The listing builds one solid part. Answer for the finished solid, in the listing's coordinates (mm). Coordinates: 2 decimals unless noted, no trailing zeros. Loops run counter-clockwise (first coordinate to the right, second up) from the corner with the lowest first, then second, coordinate; pieces in that order, holes last. Notation, with made-up numbers: M 56,54 L 66,54 A23 cw 66,71 Z; hole C 30.25,-39 d1. An arc over 180 degrees is marked long. Answer in a Markdown table with one row per item. Add a question column.
from build123d import *

# Parameters (mm, degrees)
SKETCH4_R          = 100
CUT_EXTRUDE2_DEPTH = 10
SKETCH5_R          = 250
CUT_EXTRUDE4_DEPTH = 1
SKETCH6_R          = 1.241785282
CUT_EXTRUDE5_DEPTH = 201


with BuildPart() as part:
    # Sketch1 → Revolve2 (revolve)
    with BuildSketch(Plane.XY):
        Polygon((0, 0), (0, 251), (202, 251), (202, 150), align=None)
        Polygon((201, 249.758214718), (201, 151), (0.5, 2.113861386), (1, 249.758214718), align=None, mode=Mode.SUBTRACT)
    revolve(axis=Axis((0, 251, 0), (1, 0, 0)))

    # Sketch4 → Cut-Extrude2 (cut)
    with BuildSketch(Plane(origin=(202, 0, 0), x_dir=(0, 0, -1), z_dir=(1, 0, 0))):
        with Locations((0, 251)):
            Circle(SKETCH4_R)
    extrude(amount=-CUT_EXTRUDE2_DEPTH, mode=Mode.SUBTRACT)

    # Sketch5 → Cut-Extrude4 (cut)
    with BuildSketch(Plane.ZY):
        with Locations((0, 251)):
            Circle(SKETCH5_R)
    extrude(amount=-CUT_EXTRUDE4_DEPTH, mode=Mode.SUBTRACT)

    # Sketch6 → Cut-Extrude5 (cut)
    with BuildSketch(Plane.ZY.offset(-1)):
        with Locations((0, 251)):
            Circle(SKETCH6_R)
    extrude(amount=-CUT_EXTRUDE5_DEPTH, mode=Mode.SUBTRACT)


solid = part.part
(1) A cutting plane is placed at D-D (x = 19). Give the vertices of the cut face in (y, z).
(2) Straight lines are drawn through the part: line 1 (Z direction, x = 201.8, y = 251); line 2 (Z direction, x = 201.7, y = 251); line 3 (Y direction, x = 105, z = 108.5). For each, find the intervals that lie inside material, in ascending order.
(3) A cutting plane is placed at B-B (y = 251). Give the vertices of the cut face in (x, z).
(4) A cutting plane is placed at C-C (x = 54). Give the vertices of the cut face in (y, z), plus the area to 3 significant figures.
(5) A cutting plane is placed at A-A (z = 0). Give the vertices of the cut face in (x, y), plus the area to 3 significant figures.
(6) Each of these flat-tipped pins is pushed along its axis until it touches: pin 1 (12 mm diameter, centred on x = 180, z = -14, fed in from +Y); pin 2 (5 mm diameter, centred on x = 168, y = 293, fed in from +Z); pin 3 (1 mm diameter, centred on x = 42, y = 63.5, fed in from -Z). Where does it stop, or does it pass through?
(7) The mould has two halves that part along Y. Classify faces 1 (the face through (202, 153, -23)), 2 (the face through (189.36, 361.28, -4.85)), 3 (the face through (201.51, 281.04, -95.38)): released by +Y, released by -Y, zero draft, split by the parting line, or undercut.
Solved:
| question | item | result |
|---|---|---|
| 1 | outline | C 251,0 d473.78; hole C 251,0 d470.3 |
| 2 | line 1 | z = -101.15 to -100, 100 to 101.15 |
| 2 | line 2 | z = -101.22 to -100, 100 to 101.22 |
| 2 | line 3 | y = 116.21 to 118.46, 383.54 to 385.79 |
| 3 | outline | M 0,-251 L 202,-101 L 202,-100 L 201,-100 L 1,-248.51 L 1,-250 L 0,-250 Z; M 0,250 L 1,250 L 1,248.51 L 201,100 L 202,100 L 202,101 L 0,251 Z |
| 4 | outline | C 251,0 d421.8; hole C 251,0 d418.32 |
| 4 | area | 2,300 mm² |
| 5 | outline | M 0,0 L 202,150 L 202,151 L 201,151 L 1,2.49 L 1,1 L 0,1 Z; M 0,501 L 1,501 L 1,499.51 L 201,351 L 202,351 L 202,352 L 0,502 Z |
| 5 | area | 701 mm² |
| 6 | pin 1 | stops at y = 372.03 |
| 6 | pin 2 | stops at z = 121.2 |
| 6 | pin 3 | stops at z = -115.8 |
| 7 | face 1 | zero draft |
| 7 | face 2 | split by the parting line |
| 7 | face 3 | undercut |
